The listing builds one solid part. Answer for the finished solid, in the listing's coordinates (mm). Face numbers are marked on the shaded views. Give positions to 0.01 mm unless a question says otherwise; leave off trailing zeros. Order: outer loops, then holes, each group sorted by start corner. A loop starts at its lowest first (then second) coordinate and runs counter-clockwise, first axis right, second up.
Autodesk Inventor part; units mm, degrees
ref_plane "Work Plane1" through (-21.2861, 0, 0) normal (0, -0.866, -0.5) x (1, 0, 0)
ref_plane "YZ Plane" through (0, 0, 0) normal (1, 0, 0) x (0, 1, 0)
ref_plane "XZ Plane" through (0, 0, 0) normal (0, 1, 0) x (-1, 0, 0)
sketch "Sketch1" plane through (0, 0, 0) normal (1, 0, 0) x (0, 1, 0)
  line L0 (-12.1244, 0) -> (-6.0622, 10.5)
  line L1 (-6.0622, 10.5) -> (6.0622, 10.5)
  line L2 (6.0622, 10.5) -> (12.1244, 0)
  line L3 (12.1244, 0) -> (6.0622, -10.5)
  line L4 (6.0622, -10.5) -> (-6.0622, -10.5)
  line L5 (-6.0622, -10.5) -> (-12.1244, 0)
  point P0 (0, 0)
  point P1 (0, 0)
  dimension "d0" = 24.2487
extrude "Body" add sketch "Sketch1" along normal blind 14.1
sketch "Sketch2" plane through (0, 0, 0) normal (0, 0, 1) x (1, 0, 0)
  line L0 (0, 6.0622) -> (0, 12.1244)
  line L1 (0, 12.1244) -> (14.1, 12.1244)
  line L2 (14.1, 6.0622) -> (14.1, 12.1244)
  line L3 (-2.82, 0) -> (16.92, 0)
  line L4 (1.3304, 12.1244) -> (0, 9.82)
  line L5 (12.7696, 12.1244) -> (14.1, 9.82)
  dimension "d3" = 30
  dimension "d4" = 30
  dimension "d5" = 19.64
  dimension "d6" = 19.64
revolve "Chamfer1" cut sketch "Sketch2" angle 360 about axis through (-10, 0, 0) along (1, 0, 0)
sketch "Sketch3" plane through (14.1, 0, 0) normal (1, 0, 0) x (0, 0, -1)
  arc A0 (-0.625, -1.0825) -> (0.625, -1.0825) centre (0, 0) ccw
hole "Thread" at (14.1, 0, 0) direction (-1, 0, 0) diameter 12.376 end through all
chamfer "Chamfer2" distance 0.8119 angle 30 1 edges at (14.1, 0, 6.188) measured on face at (14.1, 8.4992, -1.032)
chamfer "Chamfer3" distance 0.8119 angle 30 1 edges at (0, 0, 6.188) measured on face at (0, 8.4992, -1.032)
ref_plane "Work Plane1" through (-21.2861, 0, 0) normal (0, -0.866, -0.5) x (1, 0, 0)
equation "\"d0\" = 1.1547 * SW"
equation "\"d1\" = KOH"
equation "\"d3\" = ANG1"
equation "\"d4\" = ANG2"
equation "\"d5\" = SW0"
equation "\"d6\" = SW01"
equation "\"d8\" = -0.5 * GD1 + 0.5 * NND"
equation "\"d40\" = -0.5 * GD1 + 0.5 * NND"
equation "\"d10\" = -0.5 * GD1 + 0.5 * NND"
equation "\"d41\" = -0.5 * GD1 + 0.5 * NND"
equation "\"ANG1\" = 30deg"
equation "\"ANG2\" = 30deg"
equation "\"NND\" = 14"
equation "\"KOH\" = 14.1"
equation "\"SW\" = 21"
equation "\"SW0\" = 19.64"
equation "\"SW01\" = SW0"
equation "\"GUL\" = 0.541266 * PTC"
equation "\"THREADDIA\" = 14"
equation "\"TOA\" = 30deg"
equation "\"PTC\" = 1.5"
equation "\"E0\" = 23.36"
equation "\"GAL\" = 0.541266 * PTC"
equation "\"KOH1\" = 10.72"
properties part number "ISO 8674 - M14 x 1.5" material "Steel"
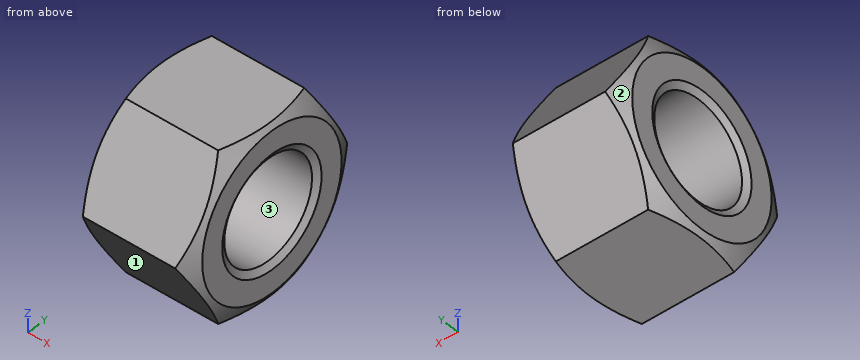
1) Find section B-B (y = 0). Write down the section's boundary in (x, z).
Geometry says:
outline: (0, -9.82) - (0.39, -10.5) - (13.71, -10.5) - (14.1, -9.82) - (14.1, -7) - (13.63, -6.19) - (0.47, -6.19) - (0, -7) - close; (0, 7) - (0.47, 6.19) - (13.63, 6.19) - (14.1, 7) - (14.1, 9.82) - (13.71, 10.5) - (0.39, 10.5) - (0, 9.82) - close
2) Given P1, Ø2, axis at x = 5.5, z = -0.5, coming from the -Y side; P2, Ø3, axis at x = 11.5, z = 4, coming from the -Y side; P3, Ø1.5, axis at x = 1.5, z = -1, coming from the +Y side, each flat-ended and moving along its own axis, determine where each tip first touches the part or whether it passes through.
Geometry says:
P1: stops at y = -12.12
P2: stops at y = -10.68
P3: stops at y = 11.98
3) Find section A-A (x = 5.75). Write down the section's boundary in (y, z), then the cut area to 3 significant figures.
Geometry says:
outline: (-12.12, 0) - (-6.06, -10.5) - (6.06, -10.5) - (12.12, 0) - (6.06, 10.5) - (-6.06, 10.5) - close; hole circle Ø12.38 at (0, 0)
area: 262 mm2
4) Straight lines are drawn through the part: probe 1 along Z at (x, y) = (8.75, 0); probe 2 along Z at (x, y) = (11, -1.5); probe 3 along Y at (x, z) = (1.75, -0.25). For each, find the intervals that lie inside material, in ascending order.
Geometry says:
probe 1: z = -10.5 to -6.19, 6.19 to 10.5
probe 2: z = -10.5 to -6, 6 to 10.5
probe 3: y = -11.98 to -6.18, 6.18 to 11.98
5) For a pull along Z with two mould halves and no side action, classify the marked faces 1, 2 and 3 as +Z half, -Z half, draft (parallel to the pull), parting line (faces both ways), or undercut.
Geometry says:
face 1: -Z half
face 2: parting line
face 3: undercut
